Check sheet for the modelled part. Datum: model origin and axes. Units: mm. A direction names the side the tool comes from. Coordinates: 2 decimals unless noted, no trailing zeros. Order: outer loops, then holes, each group sorted by start corner. A loop starts at its lowest first (then second) coordinate and runs counter-clockwise, first axis right, second up. Notation, with made-up numbers: M 72,31.5 L 89,31.5 A29 cw 89,56.5 Z; hole C -20,0 d9. An arc over 180 degrees is marked long. Answer in a Markdown table with one row per item. Add a question column.
from build123d import *

# Parameters (mm, degrees)
BASPROSKE_W     = 5
BASPROSKE_H     = 3
TOOTHCUT_DEPTH  = 7.557438524
TEETHCUTS_COUNT = 10
TEETHCUTS_ANGLE = 324
BORSKE_R        = 1
BORE_DEPTH      = 50.000762
SKETCH_1_R      = 9
SKETCH_1_R_2    = 1.5
EXTRUDE_1_DEPTH = 1
EXTRUDE_START   = 1
SKETCH_1_3_R    = 2
EXTRUDE_2_DEPTH = 5


with BuildPart() as part:
    # BasProSke → Base-Revolve (revolve)
    with BuildSketch(Plane(origin=(0, 0, 0), x_dir=(1, 0, 0), z_dir=(0, 1, 0)), mode=Mode.PRIVATE) as base_revolve_sk:
        with Locations((2.5, 1.5)):
            Rectangle(BASPROSKE_W, BASPROSKE_H)
    revolve(base_revolve_sk.sketch.rotate(Axis((-10, 0, 0), (1, 0, 0)), 180), axis=Axis((-10, 0, 0), (1, 0, 0)))

    # TooCutSke → ToothCut (cut, through all)
    with BuildSketch(Plane(origin=(0, 0, 0), x_dir=(0, 0, -1), z_dir=(1, 0, 0))):
        with BuildLine():
            ThreePointArc((0.296449938, 1.850403587), (0, 1.874), (-0.296449938, 1.850403587))
            ThreePointArc((-0.296449938, 1.850403587), (-0.428089565, 2.470295585), (-0.905889751, 2.886591228))
            ThreePointArc((-0.905889751, 2.886591228), (0, 3.0254), (0.905889751, 2.886591228))
            ThreePointArc((0.905889751, 2.886591228), (0.428089565, 2.470295585), (0.296449938, 1.850403587))
        make_face()
    toothcut = extrude(amount=TOOTHCUT_DEPTH, mode=Mode.SUBTRACT)

    # TeethCuts: ToothCut ×10 about axis
    teethcuts_axis = Axis((-10, 0, 0), (1, 0, 0))
    for i in range(1, TEETHCUTS_COUNT):
        add(toothcut.rotate(teethcuts_axis, i * TEETHCUTS_ANGLE / (TEETHCUTS_COUNT - 1)), mode=Mode.SUBTRACT)

    # BorSke → Bore (cut, symmetric)
    with BuildSketch(Plane(origin=(0, 0, 0), x_dir=(0, 0, -1), z_dir=(1, 0, 0))):
        with Locations(Location((0, 0, 0), (0, 0, 180))):
            Circle(BORSKE_R)
    extrude(amount=BORE_DEPTH, both=True, mode=Mode.SUBTRACT)

    # 草图1 → 凸台-拉伸1 (add)
    with BuildSketch(Plane.ZY):
        Circle(SKETCH_1_R)
        Circle(SKETCH_1_R_2, mode=Mode.SUBTRACT)
    extrude(amount=EXTRUDE_1_DEPTH)

    # 草图1<3> → 凸台-拉伸2 (add)
    with BuildSketch(Plane.ZY.offset(EXTRUDE_START)):
        with Locations((0, 6.25)):
            Circle(SKETCH_1_3_R)
        with Locations((-5.412658774, -3.125)):
            Circle(SKETCH_1_3_R)
        with Locations((5.412658774, -3.125)):
            Circle(SKETCH_1_3_R)
    extrude(amount=EXTRUDE_2_DEPTH)


solid = part.part
1. Go/stop test with flat-tipped pins: pin 1 Ø2 at (x, y) = (3, -3.5) entering from +Z; pin 2 Ø1.2 at (y, z) = (0, 0) entering from +X; pin 3 Ø1.5 at (y, z) = (-2, 4) entering from +X; pin 4 Ø1 at (x, y) = (0, 5) entering from +Z. Record where each tip stops, or that it passes through.
2. Section check C-C on z = 4.5. Enter the section's corners in (x, y), then the cut area to 3 significant figures.
3. Section check A-A on z = 0. Enter the section's corners in (x, y), then the cut area to 3 significant figures.
4. Release check for a two-part mould opening along Y. For faces 4 (the cylindrical face through (-3.465, 8.233, -0.26)), 5 (the flat face through (-6, 6, 0)), 6 (the cylindrical face through (2.5, -2.2, 1.1)) record: released by +Y, released by -Y, zero draft, split by the parting line, or undercut.
5. Section check D-D on x = -2.25. Enter the section's corners in (y, z) (3 decimals), then the cut area to 3 significant figures.
6. Set-up check for faces 1 (the cylindrical face through (-0.49, 0.07, -1.5)), 2 (the flat face through (0, 2.1, -0.1)), 3 (the cylindrical face through (-0.493, 8.923, -1.172)): record each of +Z, -Z, +X, -X, +Y, -Y from which the full face is reachable in a straight line by a thin tool's end or side.
7. Section check B-B on y = -3.75. Enter the section's corners in (x, z).
8. Scan lines: line 1 (Y direction, x = -0.55, z = 0); line 2 (Y direction, x = 3.2, z = 0); line 3 (X direction, y = 1, z = -0.25). Record each from-to range of solid material in increasing order.
Result sheet:
| question | item | result |
|---|---|---|
| 1 | pin 1 | z = 1.1 |
| 1 | pin 2 | through |
| 1 | pin 3 | x = 0 |
| 1 | pin 4 | z = 7.79 |
| 2 | outline | M -6,-4.9 L -1,-4.9 L -1,-7.79 L 0,-7.79 L 0,7.79 L -1,7.79 L -1,-1.35 L -6,-1.35 Z |
| 2 | area | 33.4 mm^2 |
| 3 | outline | M -6,4.25 L -1,4.25 L -1,1.5 L 0,1.5 L 0,1 L 5,1 L 5,1.87 L 0,1.87 L 0,9 L -1,9 L -1,8.25 L -6,8.25 Z; M -1,-9 L 0,-9 L 0,-1.87 L 5,-1.87 L 5,-1 L 0,-1 L 0,-1.5 L -1,-1.5 Z |
| 3 | area | 43.7 mm^2 |
| 4 | face 4 | split by the parting line |
| 4 | face 5 | zero draft |
| 4 | face 6 | undercut |
| 5 | outline | C -3.125,-5.413 d4; C -3.125,5.413 d4; C 6.25,0 d4 |
| 5 | area | 37.7 mm^2 |
| 6 | face 1 | -X |
| 6 | face 2 | +X |
| 6 | face 3 | +X, -X |
| 7 | outline | M -6,-7.31 L -1,-7.31 L -1,-8.18 L 0,-8.18 L 0,8.18 L -1,8.18 L -1,7.31 L -6,7.31 L -6,3.51 L -1,3.51 L -1,-3.51 L -6,-3.51 Z |
| 8 | line 1 | -9 to -1.5, 1.5 to 9 |
| 8 | line 2 | -1.87 to -1, 1 to 1.87 |
| 8 | line 3 | 0 to 5 |
